The listing builds one solid part. Answer for the finished solid, in the listing's coordinates (mm). Face numbers are marked on the shaded views. Coordinates: 2 decimals unless noted, no trailing zeros. Order: outer loops, then holes, each group sorted by start corner. A loop starts at its lowest first (then second) coordinate and runs counter-clockwise, first axis right, second up.
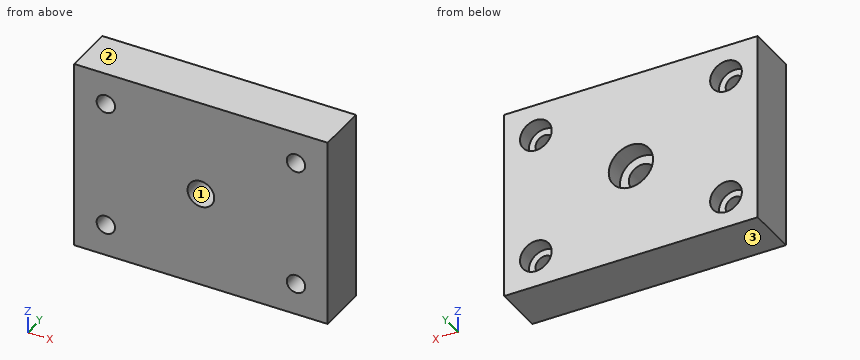
from build123d import *

# Parameters (mm, degrees)
SKETCH1_W                         = 80
SKETCH1_H                         = 60
BASE_FLANGE1_DEPTH                = 15.875
CBORE_FOR_M5_SHCS1_D              = 5.8
CBORE_FOR_M5_SHCS1_CBORE_D        = 10
CBORE_FOR_M5_SHCS1_CBORE_DEPTH    = 5
F_3_8_24_TAPPED_HOLE1_D           = 8.4328
F_3_8_24_TAPPED_HOLE1_CBORE_D     = 14
F_3_8_24_TAPPED_HOLE1_CBORE_DEPTH = 6.35


# Sheet-metal steps are written as plain solids
with BuildPart() as part:
    # Sketch1 → Base-Flange1 (new body)
    with BuildSketch(Plane(origin=(0, 0, 0), x_dir=(1, 0, 0), z_dir=(0, 1, 0))):
        Rectangle(SKETCH1_W, SKETCH1_H)
    extrude(amount=-BASE_FLANGE1_DEPTH)

    # CBORE for M5 SHCS1 (through all)
    with Locations(Plane(origin=(0, 0, 0), x_dir=(1, 0, 0), z_dir=(0, 1, 0))):
        with Locations((-30, -20), (-30, 20), (30, 20), (30, -20)):
            CounterBoreHole(CBORE_FOR_M5_SHCS1_D / 2, CBORE_FOR_M5_SHCS1_CBORE_D / 2, CBORE_FOR_M5_SHCS1_CBORE_DEPTH)

    # 3/8-24 Tapped Hole1 (through all)
    with Locations(Plane(origin=(0, 0, 0), x_dir=(1, 0, 0), z_dir=(0, 1, 0))):
        with Locations((0, 0)):
            CounterBoreHole(F_3_8_24_TAPPED_HOLE1_D / 2, F_3_8_24_TAPPED_HOLE1_CBORE_D / 2, F_3_8_24_TAPPED_HOLE1_CBORE_DEPTH)


solid = part.part
(1) Given pin 1 Ø5 at (x, z) = (-1.5, -4) entering from +Y; pin 2 Ø5 at (x, z) = (0, 0) entering from +Y; pin 3 Ø5 at (x, z) = (30.5, 22) entering from +Y, each flat-ended and moving along its own axis, determine where each tip first touches the part or whether it passes through.
(2) Find section C-C on z = 0. Determine the outline of the cut face in (x, y) (3 decimals), then the cut area to 3 significant figures.
(3) Find section B-B on y = -11. Determine the outline of the cut face in (x, z), then the cut area to 3 significant figures.
(4) Find section A-A on z = -20. Determine the outline of the cut face in (x, y) (3 decimals), then the cut area to 3 significant figures.
(5) The mould has two halves that part along Z. Classify the marked faces 1, 2 and 3: pulls with the +Z half, pulls with the -Z half, needs draft (parallel to the pull), parting line crosses it, or undercut.
(6) Find section D-D on x = 0. Determine the outline of the cut face in (y, z) (3 decimals).
(7) Find the intervals of material crossed by probe 1 along Z at (x, y) = (-30, -9.75); probe 2 along X at (y, z) = (-8.5, -20); probe 3 along Z at (x, y) = (-30, -1.8), in increasing order.
Resolved:
1. pin 1: stops at y = -6.35
1. pin 2: passes through
1. pin 3: stops at y = -5
2. outline: (-40, -15.875) - (-4.216, -15.875) - (-4.216, -6.35) - (-7, -6.35) - (-7, 0) - (-40, 0) - close; (4.216, -15.875) - (40, -15.875) - (40, 0) - (7, 0) - (7, -6.35) - (4.216, -6.35) - close
2. area: 1,100 mm2
3. outline: (-40, -30) - (40, -30) - (40, 30) - (-40, 30) - close; hole circle Ø5.8 at (-30, -20); hole circle Ø5.8 at (-30, 20); hole circle Ø8.43 at (0, 0); hole circle Ø5.8 at (30, -20); hole circle Ø5.8 at (30, 20)
3. area: 4,640 mm2
4. outline: (-40, -15.875) - (-32.9, -15.875) - (-32.9, -5) - (-35, -5) - (-35, 0) - (-40, 0) - close; (-27.1, -15.875) - (27.1, -15.875) - (27.1, -5) - (25, -5) - (25, 0) - (-25, 0) - (-25, -5) - (-27.1, -5) - close; (32.9, -15.875) - (40, -15.875) - (40, 0) - (35, 0) - (35, -5) - (32.9, -5) - close
4. area: 1,040 mm2
5. face 1: undercut
5. face 2: pulls with the +Z half
5. face 3: pulls with the -Z half
6. outline: (-15.875, -30) - (0, -30) - (0, -7) - (-6.35, -7) - (-6.35, -4.216) - (-15.875, -4.216) - close; (-15.875, 4.216) - (-6.35, 4.216) - (-6.35, 7) - (0, 7) - (0, 30) - (-15.875, 30) - close
7. probe 1: z = -30 to -22.9, -17.1 to 17.1, 22.9 to 30
7. probe 2: x = -40 to -32.9, -27.1 to 27.1, 32.9 to 40
7. probe 3: z = -30 to -25, -15 to 15, 25 to 30
